For this review, take the finished solid that the model builds, in its own axes (mm). Coordinates: 2 decimals unless noted, no trailing zeros. Loops run counter-clockwise (first coordinate to the right, second up) from the corner with the lowest first, then second, coordinate; pieces in that order, holes last.
1. Take a section at C-C, the plane z = 5. State the section outline as (x, y) points.
2. Take a section at B-B, the plane x = 0. State the section outline as (y, z) points, then the cut area to 3 significant figures.
3. To check wall thickness, follow probe 1 along X at (y, z) = (8, 0.5); probe 2 along Z at (x, y) = (14, 16); probe 3 along Y at (x, z) = (-23, 1.5). State the ranges of each line that lie inside material, in increasing order.
4. Clearance check with flat-ended pins moving along their axes: P1, Ø1.5, axis at y = 13, z = 4.5, coming from the -X side; P2, Ø6, axis at x = -21.5, y = 17, coming from the -Z side; P3, Ø1, axis at x = -2, z = 1.5, coming from the +Y side. State where each tip first meets the part, or that it passes through.
5. Take a section at A-A, the plane y = 3. State the section outline as (x, z) points.
6. Take a section at D-D, the plane y = 13.9. State the section outline as (x, z) points.
```python
from build123d import *

# Parameters (mm, degrees)
BOSS_EXTRUDE1_DEPTH = 2
SKETCH4_R           = 1.2
BOSS_EXTRUDE2_DEPTH = 7


with BuildPart() as part:
    # Sketch3 → Boss-Extrude1 (new body)
    with BuildSketch(Plane.XY):
        with BuildLine():
            Line((30.2, 0), (20.5, 0))
            ThreePointArc((20.5, 0), (0, 20.5), (-20.5, 0))
            Line((-20.5, 0), (-30.2, 0))
            ThreePointArc((-30.2, 0), (0, 30.2), (30.2, 0))
        make_face()
    extrude(amount=BOSS_EXTRUDE1_DEPTH)

    # Sketch4 → Boss-Extrude2 (add)
    with BuildSketch(Plane(origin=(0, 0, 0), x_dir=(-1, 0, 0), z_dir=(0, 0, -1))):
        with Locations((0, 27.800000001)):
            Circle(SKETCH4_R)
        with Locations((24.075506226, 13.9)):
            Circle(SKETCH4_R)
        with Locations((-24.075506226, 13.9)):
            Circle(SKETCH4_R)
    extrude(amount=-BOSS_EXTRUDE2_DEPTH)


solid = part.part
```
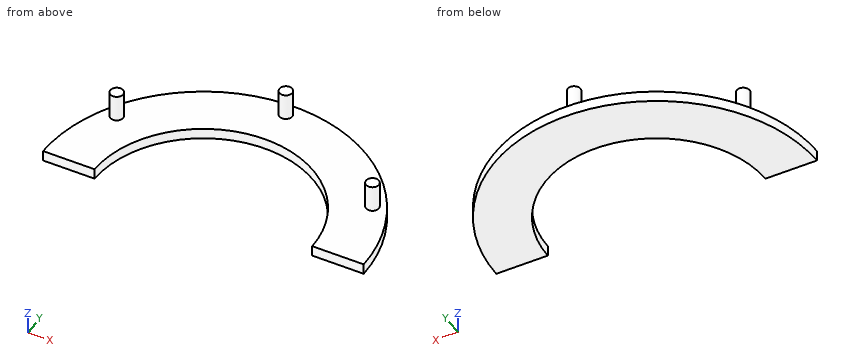
Results list:
1. outline: circle Ø2.4 at (-24.08, 13.9); circle Ø2.4 at (0, 27.8); circle Ø2.4 at (24.08, 13.9)
2. outline: (20.5, 0) - (30.2, 0) - (30.2, 2) - (29, 2) - (29, 7) - (26.6, 7) - (26.6, 2) - (20.5, 2) - close
2. area: 31.4 mm2
3. probe 1: x = -29.12 to -18.87, 18.87 to 29.12
3. probe 2: z = 0 to 2
3. probe 3: y = 0 to 19.57
4. P1: stops at x = -25.27
4. P2: stops at z = 0
4. P3: stops at y = 30.16
5. outline: (-30.05, 0) - (-20.28, 0) - (-20.28, 2) - (-30.05, 2) - close; (20.28, 0) - (30.05, 0) - (30.05, 2) - (20.28, 2) - close
6. outline: (-26.81, 0) - (-15.07, 0) - (-15.07, 2) - (-22.88, 2) - (-22.88, 7) - (-25.28, 7) - (-25.28, 2) - (-26.81, 2) - close; (15.07, 0) - (26.81, 0) - (26.81, 2) - (25.28, 2) - (25.28, 7) - (22.88, 7) - (22.88, 2) - (15.07, 2) - close
